Build history of the part. All positions in model axes, mm. Face numbers are marked on the shaded views. A direction names the side the tool comes from. Round coordinates to 2 decimals unless told otherwise and drop trailing zeros. Loops run counter-clockwise (first coordinate to the right, second up) from the corner with the lowest first, then second, coordinate; pieces in that order, holes last. Notation, with made-up numbers: (-13, 16.5) - (10, 16.5) arc R23 ccw to (10, 27.5) - close; hole circle Ø11 at (17.5, 8.25). An arc over 180 degrees is marked (long way). Use one line per item in the form item = value. Start each with the question number.
Q1. Drill centre lines: line 1 (X direction, y = 0.35, z = 40); line 2 (X direction, y = -3.25, z = 32); line 3 (X direction, y = -5.25, z = 29). Where is each one in solid material? Low to high.
Q2. Mould opens along Z. For the marked faces 3, 4 and 5 say: released by +Z, released by -Z, zero draft, split by the parting line, or undercut.
Q3. Saw through at B-B (y = -3.75). Give the cut face in (x, z) (3 decimals), then the cut area to 3 significant figures.
Q4. Saw through at A-A (z = 0). Give the cut face in (x, y), then the cut area to 3 significant figures.
Q5. Pin check, flat tips, straight feed: pin 1 (1.5 mm diameter, centred on x = 19, y = -2, fed in from +Z); pin 2 (4.5 mm diameter, centred on y = -4, z = 11.5, fed in from +X); pin 3 (1.1 mm diameter, centred on y = -0.5, z = 6.5, fed in from -X). Stop position of each tip, or through.
Q6. 3-axis set-ups, long thin cutter, end or side, ignore diameter. For the marked faces 1 and 2: which of +Z, -Z, +X, -X, +Y, -Y reach the whole face in a straight line?
Q7. Saw through at C-C (x = 20). Count the separate pieces of the cut face and the enclosed holes in it, then the cut area to 3 significant figures.
```python
from build123d import *
from build123d.topology import SkipClean

# Parameters (mm, degrees)
SKETCH1_R           = 50
SKETCH1_R_2         = 6.5
SKETCH1_W           = 76
SKETCH1_H           = 46
BOSS_EXTRUDE1_DEPTH = 1
SKETCH2_R           = 50
SKETCH2_R_2         = 48.5
BOSS_EXTRUDE2_DEPTH = 7
SKETCH3_R           = 53
SKETCH3_R_2         = 50
BOSS_EXTRUDE3_DEPTH = 2
BOSS_EXTRUDE4_START = -7
SKETCH3_2_R         = 53
SKETCH3_2_R_2       = 50
BOSS_EXTRUDE4_DEPTH = 2
SKETCH5_W           = 76
SKETCH5_H           = 46
BOSS_EXTRUDE5_DEPTH = 7
SKETCH4_W           = 80
SKETCH4_H           = 50
CUT_EXTRUDE1_DEPTH  = 2.2


with BuildPart() as part:
    # Sketch1 → Boss-Extrude1 (new, symmetric)
    with BuildSketch(Plane(origin=(0, 0, 0), x_dir=(1, 0, 0), z_dir=(0, 1, 0))):
        with Locations(Location((0, 0, 0), (0, 0, 270))):
            Circle(SKETCH1_R)
        with Locations(Location((0, 40, 0), (0, 0, 270))):
            Circle(SKETCH1_R_2, mode=Mode.SUBTRACT)
        with Locations(Location((0, -40, 0), (0, 0, 270))):
            Circle(SKETCH1_R_2, mode=Mode.SUBTRACT)
        with Locations(Location((20, -34.641016151, 0), (0, 0, 270))):
            Circle(SKETCH1_R_2, mode=Mode.SUBTRACT)
        with Locations(Location((-20, -34.641016151, 0), (0, 0, 270))):
            Circle(SKETCH1_R_2, mode=Mode.SUBTRACT)
        Rectangle(SKETCH1_W, SKETCH1_H, mode=Mode.SUBTRACT)
    extrude(amount=BOSS_EXTRUDE1_DEPTH, both=True)

    # Sketch2 → Boss-Extrude2 (add)
    with SkipClean():  # the faces are left unmerged after this step: merging them gives an invalid solid
        with BuildSketch(Plane.XZ.offset(1)):
            with Locations(Location((0, 0, 0), (0, 0, 270))):
                Circle(SKETCH2_R)
            with Locations(Location((0, 0, 0), (0, 0, 270))):
                Circle(SKETCH2_R_2, mode=Mode.SUBTRACT)
        extrude(amount=BOSS_EXTRUDE2_DEPTH)

    # Sketch3 → Boss-Extrude3 (add)
    with BuildSketch(Plane(origin=(0, 1, 0), x_dir=(1, 0, 0), z_dir=(0, 1, 0))):
        with Locations(Location((0, 0, 0), (0, 0, 270))):
            Circle(SKETCH3_R)
        with Locations(Location((0, 0, 0), (0, 0, 90))):
            Circle(SKETCH3_R_2, mode=Mode.SUBTRACT)
    extrude(amount=-BOSS_EXTRUDE3_DEPTH)

    # Sketch3<2> → Boss-Extrude4 (add)
    with BuildSketch(Plane(origin=(0, 1, 0), x_dir=(1, 0, 0), z_dir=(0, 1, 0)).offset(BOSS_EXTRUDE4_START)):
        with Locations(Location((0, 0, 0), (0, 0, 270))):
            Circle(SKETCH3_2_R)
        with Locations(Location((0, 0, 0), (0, 0, 90))):
            Circle(SKETCH3_2_R_2, mode=Mode.SUBTRACT)
    extrude(amount=-BOSS_EXTRUDE4_DEPTH)

    # Sketch5 → Boss-Extrude5 (add, through all)
    with BuildSketch(Plane.XZ.offset(1)):
        with BuildLine():
            ThreePointArc((29.876545638, 38.205261689), (21.320536736, 24.224386047), (9.54648854, 35.627980267))
            ThreePointArc((9.54648854, 35.627980267), (0, 29.5), (-9.54648854, 35.627980267))
            ThreePointArc((-9.54648854, 35.627980267), (-21.320536736, 24.224386047), (-29.876545638, 38.205261689))
            ThreePointArc((-29.876545638, 38.205261689), (-46.847402575, -12.552723687), (-6.771216656, -48.025))
            ThreePointArc((-6.771216656, -48.025), (0, -29.5), (6.771216656, -48.025))
            ThreePointArc((6.771216656, -48.025), (46.847402575, -12.552723687), (29.876545638, 38.205261689))
        make_face()
        Rectangle(SKETCH5_W, SKETCH5_H, mode=Mode.SUBTRACT)
    extrude(amount=BOSS_EXTRUDE5_DEPTH)

    # Sketch4 → Cut-Extrude1 (cut)
    with BuildSketch(Plane(origin=(0, 0, 0), x_dir=(1, 0, 0), z_dir=(0, 1, 0))):
        Rectangle(SKETCH4_W, SKETCH4_H)
    extrude(amount=-CUT_EXTRUDE1_DEPTH, mode=Mode.SUBTRACT)


solid = part.part
```
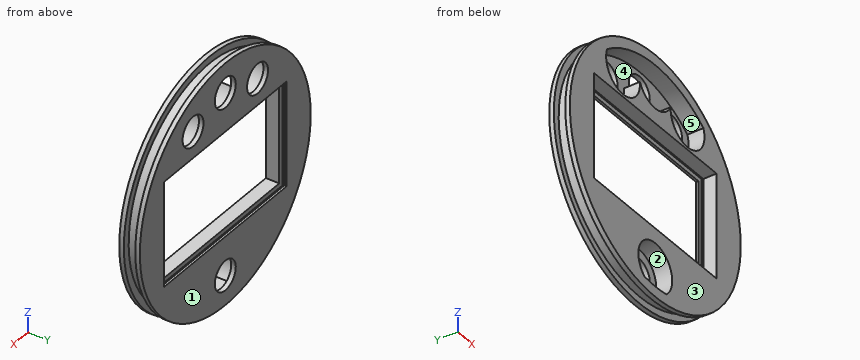
Report:
q1.line_1 = -34.77 to -23.68, -16.32 to -6.5, 6.5 to 16.32, 23.68 to 34.77
q1.line_2 = -38.42 to -30.16, -9.84 to -6.8, 6.8 to 9.84, 30.16 to 38.42
q1.line_3 = -40.73 to -28.86, -11.14 to 11.14, 28.86 to 40.73
q2.face_3 = zero draft
q2.face_4 = undercut
q2.face_5 = undercut
q3.outline = circle Ø100 at (0, 0); hole (-38, -23) - (38, -23) - (38, 23) - (-38, 23) - close; hole (-29.877, 38.205) arc R10.5 ccw (long way) to (-9.546, 35.628) arc R10.5 ccw to (9.546, 35.628) arc R10.5 ccw (long way) to (29.877, 38.205) arc R48.5 ccw to start; hole (-6.771, -48.025) arc R48.5 ccw to (6.771, -48.025) arc R10.5 ccw (long way) to start
q3.area = 2,980 mm²
q4.outline = (-53, -8) - (-38, -8) - (-38, -2.2) - (-40, -2.2) - (-40, 0) - (-38, 0) - (-38, 1) - (-53, 1) - (-53, -1) - (-50, -1) - (-50, -6) - (-53, -6) - close; (38, -8) - (53, -8) - (53, -6) - (50, -6) - (50, -1) - (53, -1) - (53, 1) - (38, 1) - (38, 0) - (40, 0) - (40, -2.2) - (38, -2.2) - close
q4.area = 231 mm²
q5.pin_1 = 46.55
q5.pin_2 = 51.96
q5.pin_3 = -52.66
q6.face_1 = +Z, -Z, +X, -X, +Y
q6.face_2 = -Y
q7.separate_pieces = 4
q7.enclosed_holes = 0
q7.area = 263 mm²
